Geometry: see drawing. Coordinates: mm, zero at the bounding-box minimum. A direction names the side the tool comes from. Coordinates: 2 decimals unless noted, no trailing zeros. Loops run counter-clockwise (first coordinate to the right, second up) from the corner with the lowest first, then second, coordinate; pieces in that order, holes last. Notation, with made-up numbers: (-36, 48) - (-6, 48) arc R12 cw to (-6, 63) - close; hole circle Ø4 at (-29, 42.5). An arc over 180 degrees is marked (long way). Use a Markdown table: item, result. Add a question column.
1. Contact query for flat-ended pins moving along their axis: P1, Ø15.5, axis at x = 32, z = 16.5, coming from the +Y side; P2, Ø8, axis at x = 12, z = 20.5, coming from the +Y side (3 decimals); P3, Ø5.5, axis at x = 22.225, y = 34.925, coming from the +Z side. Output: stop coordinate, or through.
2. Section query A-A on z = 19.05. State how many separate pieces and enclosed holes the cut face has, then the cut area to 3 significant figures.
3. Ray query, L1, parallel to X at y = 4, z = 19; L2, parallel to Z at x = 9, y = 40; L3, parallel to X at y = 36, z = 2.5. Return the intervals inside material, ascending. Write a range as [from, to].
4. Draft query along X for the marked faces 1, 2, 3 and 4. Return one class per face: released by +X, released by -X, zero draft, split by the parting line, or undercut.
5. Section query B-B on y = 30. Return the cut outline in (x, z).
6. Access query for the marked faces 5 and 6. Directions: +Z, -Z, +X, -X, +Y, -Y. A direction counts if a zero-diameter tool reaches every point of the face in a straight line with its end or side. Return the directions, or none.
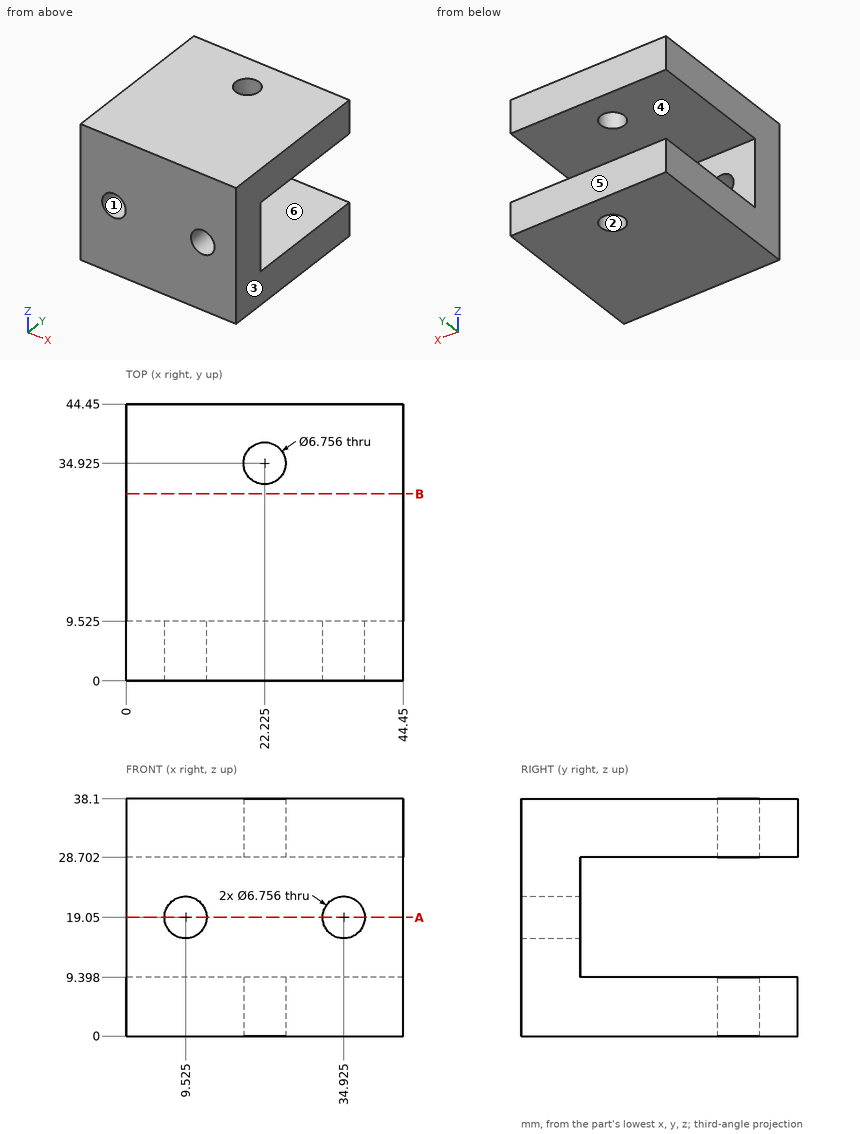
Resolved:
| question | item | result |
|---|---|---|
| 1 | P1 | y = 44.45 |
| 1 | P2 | y = 9.525 |
| 1 | P3 | through |
| 2 | separate pieces | 3 |
| 2 | enclosed holes | 0 |
| 2 | area | 295 mm² |
| 3 | L1 | [0, 6.15], [12.9, 31.55], [38.3, 44.45] |
| 3 | L2 | [0, 9.4], [28.7, 38.1] |
| 3 | L3 | [0, 19.02], [25.43, 44.45] |
| 4 | face 1 | undercut |
| 4 | face 2 | undercut |
| 4 | face 3 | released by +X |
| 4 | face 4 | zero draft |
| 5 | outline | (0, 0) - (44.45, 0) - (44.45, 9.4) - (0, 9.4) - close; (0, 28.7) - (44.45, 28.7) - (44.45, 38.1) - (0, 38.1) - close |
| 6 | face 5 | +Z, -Z, +X, -X, +Y |
| 6 | face 6 | +X, -X, +Y |
